Design review of the part built by this model. Coordinates are the model's own, in mm. A direction names the side the tool comes from. Give positions to 0.01 mm unless a question says otherwise; leave off trailing zeros. Loops run counter-clockwise (first coordinate to the right, second up) from the corner with the lowest first, then second, coordinate; pieces in that order, holes last. Notation, with made-up numbers: (79.25, 53.5) -> (126.25, 53.5) arc R14 ccw to (126.25, 71.5) -> close; hole circle Ø3 at (63.25, 61). An arc over 180 degrees is marked (long way). Answer in a Markdown table with one row per item. Add a question column.
(1) Draft analysis for pull direction X (two halves, no side actions). For faces 1 (the cylindrical face through (0.03, 4.37, 2.85)), 2 (the flat face through (-12.547, -3, 7)), 3 (the cylindrical face through (10.442, -20.278, -24.504)), 4 (the flat face through (-1.5, 7.275, 32.1)), state which applies: +X half, -X half, draft (parallel to the pull), parting line (faces both ways), or undercut.
(2) For line 1 (X direction, y = 12.5, z = -2.5); line 2 (X direction, y = -21.1, z = -13); line 3 (X direction, y = 15, z = -2), list the stretches that pass through material, from the lowest coordinate up.
(3) Consider section A-A on y = -6. Write out the cut boundary in (x, z).
(4) Consider section D-D on z = 3.6. Write out the cut boundary in (x, y) (3 decimals), then the cut area to 3 significant figures.
(5) For faces 5 (the cylindrical face through (1.05, -21.26, -16.66)), 6 (the flat face through (2.98, -19.26, -15.9)), 7 (the flat face through (0, -5, 6)), 8 (the flat face through (0, -20, 0)), 9 (the cylindrical face through (5.8, 12.34, 34.05)), list the 3-axis set-ups (+Z, -Z, +X, -X, +Y, -Y) from which the entire face can be reached by the end or side of a thin tool; tool diameter is ignored.
(6) Consider section C-C on x = 0. Count the separate pieces of the cut face and the enclosed holes in it, then the cut area to 3 significant figures.
(7) Consider section B-B on z = 10. Write out the cut boundary in (x, y) (3 decimals), then the cut area to 3 significant figures.
(8) For pin 1 (0.5 mm diameter, centred on x = 0, z = 30, fed in from -Y) (3 decimals); pin 2 (1.1 mm diameter, centred on y = -11, z = 29, fed in from -X); pin 3 (2.5 mm diameter, centred on x = 2, z = 4, fed in from +Y) (3 decimals); pin 4 (5.5 mm diameter, centred on x = -0.5, z = 32, fed in from +Y) (3 decimals), all flat-tipped, find the tip position at first contact; note any pin that passes through.
from build123d import *
from OCP.BRepFilletAPI import BRepFilletAPI_MakeChamfer

# Parameters (mm, degrees)
SKETCH4_W                = 12.46
SKETCH4_H                = 17.25
BOSS_EXTRUDE3_DEPTH      = 6
BOSS_EXTRUDE6_DEPTH      = 8.3
BOSS_EXTRUDE6_DEPTH_BACK = 17.25
SKETCH8_R                = 12.546781182
SKETCH8_R_2              = 11.15
BOSS_EXTRUDE4_DEPTH      = 17.25
SKETCH6_R                = 0.75
CUT_EXTRUDE1_DEPTH       = 5
CHAMFER1_SIZE            = 0.5
CHAMFER1_SIZE2           = 0.866025404
SKETCH10_W               = 12.46
SKETCH10_H               = 23.7
CUT_EXTRUDE3_DEPTH       = 17.25
BOSS_EXTRUDE7_START      = -8.3
BOSS_EXTRUDE7_DEPTH      = 8.3
BOSS_EXTRUDE9_START      = 10
BOSS_EXTRUDE9_DEPTH      = 10
BOSS_EXTRUDE11_START     = -8.3
SKETCH20_R               = 11.15
SKETCH20_R_2             = 7.15
BOSS_EXTRUDE11_DEPTH     = 8.3
CUT_EXTRUDE7_START       = -1.3
SKETCH21_R               = 10.15
SKETCH21_R_2             = 7.15
CUT_EXTRUDE7_DEPTH       = 1.3
CUT_EXTRUDE4_REACH       = 39.061
SKETCH11_W               = 10
SKETCH11_H               = 2
CUT_EXTRUDE8_REACH       = 54.194
SKETCH24_W               = 12.46
SKETCH24_H               = 6
BOSS_EXTRUDE10_DEPTH     = 25.093562364
SKETCH18_W               = 21.5
SKETCH18_H               = 12.438292938
CUT_EXTRUDE5_DEPTH       = 2
CUT_EXTRUDE6_DEPTH       = 58.154608998
CUT_EXTRUDE6_DEPTH_BACK  = 58.154608998
SKETCH19_R               = 3.5
FILLET1_R                = 7
SKETCH22_R               = 6.5
BOSS_EXTRUDE12_DEPTH     = 5
SKETCH23_R               = 6.075
BOSS_EXTRUDE13_DEPTH     = 5
FILLET2_R                = 1
BOSS_EXTRUDE15_DEPTH     = 2
CUT_EXTRUDE9_REACH       = 60.657
SKETCH26_R               = 0.75
CUT_EXTRUDE10_DEPTH      = 50.271969555
SKETCH28_R               = 2.1
SKETCH28_R_2             = 2.45
CUT_EXTRUDE11_DEPTH      = 7
FILLET3_R                = 1


with BuildPart() as part:
    # Sketch4 → Boss-Extrude3 (new body)
    with BuildSketch(Plane.XY):
        with Locations((0, -1.35)):
            Rectangle(SKETCH4_W, SKETCH4_H)
    extrude(amount=BOSS_EXTRUDE3_DEPTH)



with BuildPart() as body_2:
    # Sketch8 → Boss-Extrude6 (new, two sides: drawn at the far end of the back side and taken through both)
    with BuildSketch(Plane(origin=(0, -9.975, 0), x_dir=(-1, 0, 0), z_dir=(0, -1, 0)).offset(-BOSS_EXTRUDE6_DEPTH_BACK)):
        with Locations(Location((0, -23.55, 0), (0, 0, 90))):
            Circle(SKETCH8_R)
        with Locations(Location((0, -23.55, 0), (0, 0, 90))):
            Circle(SKETCH8_R_2, mode=Mode.SUBTRACT)
    extrude(amount=BOSS_EXTRUDE6_DEPTH + BOSS_EXTRUDE6_DEPTH_BACK)


with BuildPart() as part_1:
    add(part.part)

    add(body_2.part)  # Boss-Extrude4 merges body 2
    # Sketch5 → Boss-Extrude4 (add)
    with BuildSketch(Plane(origin=(0, 7.275, 0), x_dir=(1, 0, 0), z_dir=(0, 1, 0))):
        with BuildLine():
            Line((12.546781182, -23.55), (12.546781182, 0))
            Line((12.546781182, 0), (6.23, 0))
            Line((6.23, 0), (6.23, -29.7))
            Line((6.23, -29.7), (-6.23, -29.7))
            Line((-6.23, -29.7), (-6.23, 0))
            Line((-6.23, 0), (-12.546781182, 0))
            Line((-12.546781182, 0), (-12.546781182, -23.55))
            ThreePointArc((-12.546781182, -23.55), (0, -36.096781182), (12.546781182, -23.55))
        make_face()
    extrude(amount=-BOSS_EXTRUDE4_DEPTH)

    # Sketch6 → Cut-Extrude1 (cut)
    with BuildSketch(Plane(origin=(0, 7.275, 0), x_dir=(1, 0, 0), z_dir=(0, 1, 0))):
        with Locations(Location((0, -3.6, 0), (0, 0, 270))):
            Circle(SKETCH6_R)
        with Locations(Location((0, -32.1, 0), (0, 0, 270))):
            Circle(SKETCH6_R)
    extrude(amount=-CUT_EXTRUDE1_DEPTH, mode=Mode.SUBTRACT)

    # Chamfer1: one chamfer whose edges measure the first distance from different faces: ONE call of the kernel's chamfer builder (chamfer() names one face for all edges)
    chamfer1_edges_1 = [part_1.edges().sort_by_distance(p)[0] for p in [
        (0, 7.275, 2.85),
    ]]
    chamfer1_side_1 = [part_1.faces().sort_by_distance(p)[0] for p in [
        (12.202646125, 7.275, 11.775),
    ]]
    chamfer1_edges_2 = [part_1.edges().sort_by_distance(p)[0] for p in [
        (0, 7.275, 31.35),
    ]]
    chamfer1_side_2 = [part_1.faces().sort_by_distance(p)[0] for p in [
        (6.532214051, 7.275, 22.001429951),
    ]]
    chamfer1 = BRepFilletAPI_MakeChamfer(part_1.part.solid().wrapped)
    for e in chamfer1_edges_1:
        chamfer1.Add(CHAMFER1_SIZE, CHAMFER1_SIZE2, e.wrapped, chamfer1_side_1[0].wrapped)  # the first distance lies on this face
    for e in chamfer1_edges_2:
        chamfer1.Add(CHAMFER1_SIZE, CHAMFER1_SIZE2, e.wrapped, chamfer1_side_2[0].wrapped)  # the first distance lies on this face
    add(Compound.cast(chamfer1.Shape()), mode=Mode.REPLACE)

    # Sketch10 → Cut-Extrude3 (cut)
    with BuildSketch(Plane(origin=(0, 7.275, 0), x_dir=(1, 0, 0), z_dir=(0, 1, 0))):
        with Locations((0, -17.85)):
            Rectangle(SKETCH10_W, SKETCH10_H)
    extrude(amount=-CUT_EXTRUDE3_DEPTH, mode=Mode.SUBTRACT)

    # Sketch13 → Boss-Extrude7 (add)
    with BuildSketch(Plane.XZ.offset(18.275).offset(BOSS_EXTRUDE7_START)):
        with BuildLine():
            Line((-12.546781182, 23.55), (-12.546781182, 0))
            Line((-12.546781182, 0), (12.546781182, 0))
            Line((12.546781182, 0), (12.546781182, 23.55))
            ThreePointArc((12.546781182, 23.55), (0, 11.003218818), (-12.546781182, 23.55))
        make_face()
    extrude(amount=BOSS_EXTRUDE7_DEPTH)

    # Sketch15 → Boss-Extrude9 (add)
    with BuildSketch(Plane(origin=(0, 7.275, 0), x_dir=(1, 0, 0), z_dir=(0, 1, 0)).offset(BOSS_EXTRUDE9_START)):
        with BuildLine():
            Line((-12.546781182, 0), (12.546781182, 0))
            Line((12.546781182, 0), (12.546781182, -23.55))
            ThreePointArc((12.546781182, -23.55), (0, -36.096781182), (-12.546781182, -23.55))
            Line((-12.546781182, -23.55), (-12.546781182, 0))
        make_face()
        with BuildLine():
            Line((-6.23, -0.8), (6.23, -0.8))
            Line((6.23, -0.8), (6.23, -33))
            ThreePointArc((6.23, -33), (5.790660172, -34.060660172), (4.73, -34.5))
            Line((4.73, -34.5), (-4.73, -34.5))
            ThreePointArc((-4.73, -34.5), (-5.790660172, -34.060660172), (-6.23, -33))
            Line((-6.23, -33), (-6.23, -0.8))
        make_face(mode=Mode.SUBTRACT)
    extrude(amount=-BOSS_EXTRUDE9_DEPTH)

    # Sketch20 → Boss-Extrude11 (add)
    with BuildSketch(Plane.XZ.offset(18.275).offset(BOSS_EXTRUDE11_START)):
        with Locations((0, 23.55)):
            Circle(SKETCH20_R)
        with Locations(Location((0, 23.55, 0), (0, 0, 270))):
            Circle(SKETCH20_R_2, mode=Mode.SUBTRACT)
    extrude(amount=BOSS_EXTRUDE11_DEPTH)

    # Sketch21 → Cut-Extrude7 (cut)
    with BuildSketch(Plane.XZ.offset(18.275).offset(CUT_EXTRUDE7_START)):
        with Locations(Location((0, 23.55, 0), (0, 0, 270))):
            Circle(SKETCH21_R)
        with Locations(Location((0, 23.55, 0), (0, 0, 270))):
            Circle(SKETCH21_R_2, mode=Mode.SUBTRACT)
    extrude(amount=CUT_EXTRUDE7_DEPTH, mode=Mode.SUBTRACT)

    # Cut-Extrude4: up to this face of the body (flat: up to its plane)
    cut_extrude4_end = Plane(part_1.part.faces().sort_by_distance((0, -1.35, 6))[0])
    # Sketch11 → Cut-Extrude4 (cut, up to the picked face)
    with BuildSketch(Plane.XY.offset(29.7), mode=Mode.PRIVATE) as cut_extrude4_sk1:
        with Locations((0, -10.975)):
            Rectangle(SKETCH11_W, SKETCH11_H)
    cut_extrude4_tool1 = split(extrude(cut_extrude4_sk1.sketch, amount=-CUT_EXTRUDE4_REACH, mode=Mode.PRIVATE), bisect_by=cut_extrude4_end, keep=Keep.BOTH, mode=Mode.PRIVATE)
    add(cut_extrude4_tool1.solids().sort_by(Axis((0, -10.975, 29.7), (0, 0, -1)))[0], mode=Mode.SUBTRACT)

    # Sketch24 → Cut-Extrude8 (cut, up to next)
    with BuildSketch(Plane.XZ.offset(18.275), mode=Mode.PRIVATE) as cut_extrude8_sk1:
        with Locations((0, 9)):
            Rectangle(SKETCH24_W, SKETCH24_H)
    cut_extrude8_tool1 = extrude(cut_extrude8_sk1.sketch, amount=-CUT_EXTRUDE8_REACH, mode=Mode.PRIVATE) & part_1.part
    add(cut_extrude8_tool1.solids().sort_by_distance((0, -18.275, 9))[0], mode=Mode.SUBTRACT)

    # Sketch17 → Boss-Extrude10 (add)
    with BuildSketch(Plane(origin=(-12.546781182, 4.728218818, 0), x_dir=(0, -1, 0), z_dir=(1, 0, 0))):
        Polygon((26.978218818, 26.5), (26.978218818, 0), (-17.521781182, 0), (-17.521781182, 26.5), (-13.521781182, 26.5), (-13.521781182, 5), (22.978218818, 5), (22.978218818, 26.5), align=None)
    extrude(amount=BOSS_EXTRUDE10_DEPTH)

    # Sketch18 → Cut-Extrude5 (cut)
    with BuildSketch(Plane.ZX.offset(-18.25)):
        with Locations((-15.75, 0)):
            Rectangle(SKETCH18_W, SKETCH18_H)
    extrude(amount=-CUT_EXTRUDE5_DEPTH, mode=Mode.SUBTRACT)

    # Sketch19 → Cut-Extrude6 (cut, two sides: drawn at the far end of the back side and taken through both)
    with BuildSketch(Plane.ZX.offset(-20.25).offset(-CUT_EXTRUDE6_DEPTH_BACK)):
        with Locations((-20, 0)):
            Circle(SKETCH19_R)
    extrude(amount=CUT_EXTRUDE6_DEPTH + CUT_EXTRUDE6_DEPTH_BACK, mode=Mode.SUBTRACT)

    # Fillet1
    fillet1_edges = [part_1.edges().sort_by_distance(p)[0] for p in [
        (12.546781182, -20.25, -26.5),
        (-12.546781182, -20.25, -26.5),
        (12.546781182, 20.25, -26.5),
        (-12.546781182, 20.25, -26.5),
    ]]
    fillet(fillet1_edges, radius=FILLET1_R)

    # Sketch22 → Boss-Extrude12 (add)
    with BuildSketch(Plane(origin=(0, 22.25, 0), x_dir=(1, 0, 0), z_dir=(0, 1, 0))):
        with Locations(Location((0, 20, 0), (0, 0, 270))):
            Circle(SKETCH22_R)
    extrude(amount=-BOSS_EXTRUDE12_DEPTH)

    # Sketch23 → Boss-Extrude13 (add)
    with BuildSketch(Plane.XZ.offset(-17.25)):
        with Locations(Location((0, -20, 0), (0, 0, 270))):
            Circle(SKETCH23_R)
    extrude(amount=BOSS_EXTRUDE13_DEPTH)

    # Fillet2
    fillet2_edges = [part_1.edges().sort_by_distance(p)[0] for p in [
        (0, 12.25, -13.925),
    ]]
    fillet(fillet2_edges, radius=FILLET2_R)

    # Sketch25 → Boss-Extrude15 (add)
    with BuildSketch(Plane(origin=(0, -20.25, 0), x_dir=(1, 0, 0), z_dir=(0, 1, 0))):
        Polygon((-6.219146469, 5), (-2.5, 5), (-3.1585, 20), (-3.44385, 26.5), (-6.219146469, 26.5), align=None)
        Polygon((6.219146469, 5), (2.5, 5), (3.1585, 20), (3.44385, 26.5), (6.219146469, 26.5), align=None)
    extrude(amount=BOSS_EXTRUDE15_DEPTH)

    # Sketch26 → Cut-Extrude9 (cut, up to next)
    with BuildSketch(Plane(origin=(0, -22.25, 0), x_dir=(-1, 0, 0), z_dir=(0, -1, 0)), mode=Mode.PRIVATE) as cut_extrude9_sk1:
        with Locations(Location((0, 10, 0), (0, 0, 90))):
            Circle(SKETCH26_R)
    cut_extrude9_tool1 = extrude(cut_extrude9_sk1.sketch, amount=-CUT_EXTRUDE9_REACH, mode=Mode.PRIVATE) & part_1.part
    # Sketch26 → Cut-Extrude9 (cut, up to next)
    with BuildSketch(Plane(origin=(0, -22.25, 0), x_dir=(-1, 0, 0), z_dir=(0, -1, 0)), mode=Mode.PRIVATE) as cut_extrude9_sk2:
        with Locations(Location((0, 13, 0), (0, 0, 90))):
            Circle(SKETCH26_R)
    cut_extrude9_tool2 = extrude(cut_extrude9_sk2.sketch, amount=-CUT_EXTRUDE9_REACH, mode=Mode.PRIVATE) & part_1.part
    # Sketch26 → Cut-Extrude9 (cut, up to next)
    with BuildSketch(Plane(origin=(0, -22.25, 0), x_dir=(-1, 0, 0), z_dir=(0, -1, 0)), mode=Mode.PRIVATE) as cut_extrude9_sk3:
        with Locations(Location((0, 7.5, 0), (0, 0, 90))):
            Circle(SKETCH26_R)
    cut_extrude9_tool3 = extrude(cut_extrude9_sk3.sketch, amount=-CUT_EXTRUDE9_REACH, mode=Mode.PRIVATE) & part_1.part
    add(cut_extrude9_tool1.solids().sort_by_distance((0, -22.25, -10))[0], mode=Mode.SUBTRACT)
    add(cut_extrude9_tool2.solids().sort_by_distance((0, -22.25, -13))[0], mode=Mode.SUBTRACT)
    add(cut_extrude9_tool3.solids().sort_by_distance((0, -22.25, -7.5))[0], mode=Mode.SUBTRACT)

    # Sketch27 → Cut-Extrude10 (cut, through all)
    with BuildSketch(Plane.ZY.offset(12.546781182)):
        Polygon((-26.5, 22.25), (0, 22.25), (0, 17.275), (-10.361855954, 17.275), (-10.361855954, 7.850012942), (-26.5, 7.850012942), align=None)
    extrude(amount=-CUT_EXTRUDE10_DEPTH, mode=Mode.SUBTRACT)

    # Sketch28 → Cut-Extrude11 (cut)
    with BuildSketch(Plane(origin=(0, 17.275, 0), x_dir=(1, 0, 0), z_dir=(0, 1, 0))):
        with Locations(Location((-8, 2.5, 0), (0, 0, 270))):
            Circle(SKETCH28_R)
        with Locations(Location((8, 2.5, 0), (0, 0, 270))):
            Circle(SKETCH28_R)
        with Locations(Location((0, 2.5, 0), (0, 0, 270))):
            Circle(SKETCH28_R_2)
    extrude(amount=-CUT_EXTRUDE11_DEPTH, mode=Mode.SUBTRACT)

    # Fillet3
    # the kernel refuses this fillet: 1 mm, written as the material it takes off along each edge
    with BuildSketch(Plane(origin=(-8, 17.275, -2.5), x_dir=(0, 0, 1), z_dir=(-1, 0, 0))) as fillet3_piece_1:
        with BuildLine():
            CenterArc((2.1 + FILLET3_R, -FILLET3_R), FILLET3_R, 90, 90)
            Line((2.1, -FILLET3_R), (2.1, 0))
            Line((2.1, 0), (2.1 + FILLET3_R, 0))
        make_face()
    revolve(axis=Axis((-8, 17.275, -2.5), (0, 1, 0)), mode=Mode.SUBTRACT)
    with BuildSketch(Plane(origin=(8, 17.275, -2.5), x_dir=(0, 0, 1), z_dir=(-1, 0, 0))) as fillet3_piece_2:
        with BuildLine():
            CenterArc((2.1 + FILLET3_R, -FILLET3_R), FILLET3_R, 90, 90)
            Line((2.1, -FILLET3_R), (2.1, 0))
            Line((2.1, 0), (2.1 + FILLET3_R, 0))
        make_face()
    revolve(axis=Axis((8, 17.275, -2.5), (0, 1, 0)), mode=Mode.SUBTRACT)


solid = part_1.part
Values follow:
| question | item | result |
|---|---|---|
| 1 | face 1 | undercut |
| 1 | face 2 | -X half |
| 1 | face 3 | +X half |
| 1 | face 4 | undercut |
| 2 | line 1 | -12.55 to -10.1, -5.9 to -2.45, 2.45 to 5.9, 10.1 to 12.55 |
| 2 | line 2 | -12.55 to -0.75, 0.75 to 12.55 |
| 2 | line 3 | -12.55 to -10.04, -5.96 to -2.4, 2.4 to 5.96, 10.04 to 12.55 |
| 3 | outline | (-12.55, -5) -> (12.55, -5) -> (12.55, 23.55) arc R12.55 ccw to (-12.55, 23.55) -> close; hole (-6.23, 6) -> (6.23, 6) -> (6.23, 29.7) -> (-6.23, 29.7) -> close |
| 4 | outline | (-12.547, -18.275) -> (12.547, -18.275) -> (12.547, 17.275) -> (6.23, 17.275) -> (6.23, 7.275) -> (1.25, 7.275) -> (0.75, 6.409) -> (0.75, 2.275) -> (-0.75, 2.275) -> (-0.75, 6.409) -> (-1.25, 7.275) -> (-6.23, 7.275) -> (-6.23, 17.275) -> (-12.547, 17.275) -> close |
| 4 | area | 760 mm2 |
| 5 | face 5 | -Y |
| 5 | face 6 | -Z, +Y |
| 5 | face 7 | +Y, -Y |
| 5 | face 8 | +Z, +X, -X, -Y |
| 5 | face 9 | +Y |
| 6 | separate pieces | 7 |
| 6 | enclosed holes | 0 |
| 6 | area | 520 mm2 |
| 7 | outline | (-12.547, -18.275) -> (-6.23, -18.275) -> (-6.23, 17.275) -> (-12.547, 17.275) -> close; (6.23, -18.275) -> (12.547, -18.275) -> (12.547, 17.275) -> (6.23, 17.275) -> close |
| 7 | area | 449 mm2 |
| 8 | pin 1 | y = -9.975 |
| 8 | pin 2 | x = -11.55 |
| 8 | pin 3 | y = 7.275 |
| 8 | pin 4 | y = 17.275 |
